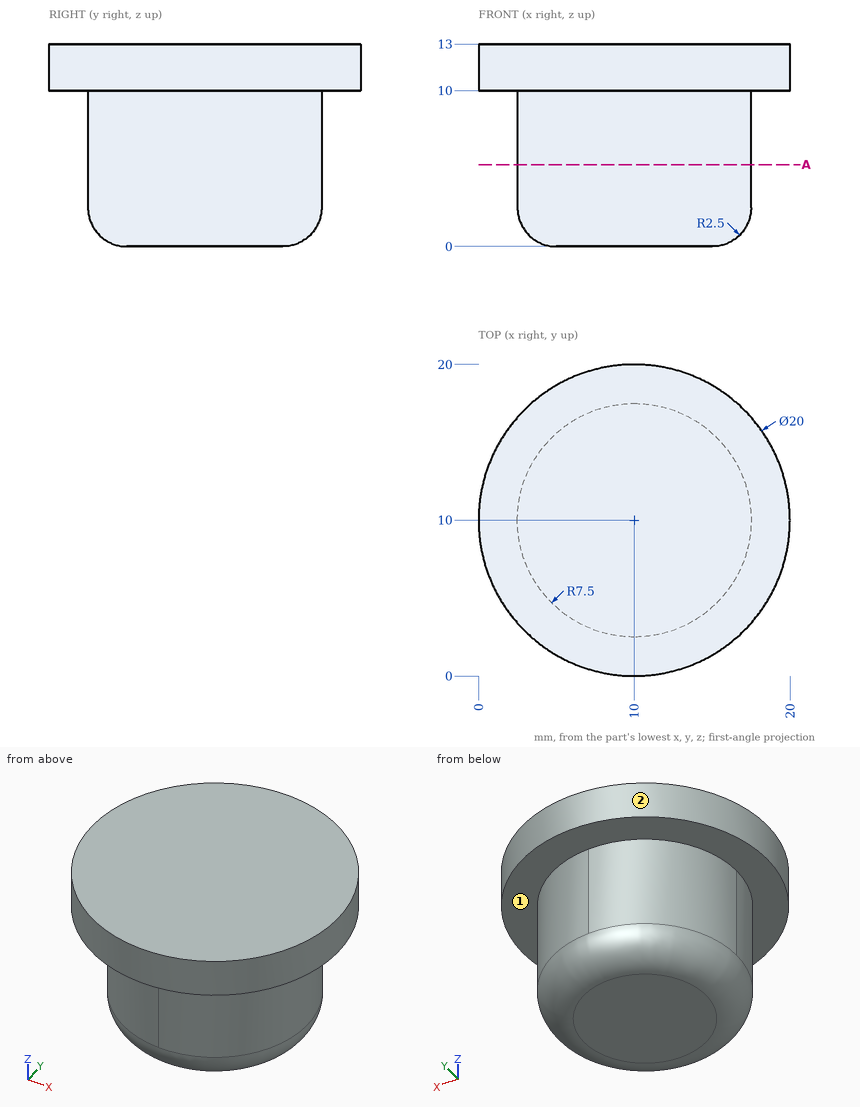
Job drawing, mm, ordinate dimensions from the low corner. One solid piece. A direction names the side the tool comes from. Coordinates: 2 decimals unless noted, no trailing zeros. Write each loop counter-clockwise with the first axis right and the second up, starting at its lowest first coordinate (ties: lowest second). Pieces come first, ordered by that corner, then holes.
Item 1: Which spindle directions (+Z, -Z, +X, -X, +Y, -Y) get a long thin tool onto all of the face, cutting with end or side? Do the marked faces 1 and 2. Say none if no direction does.
Item 2: Probe line 1 (Z direction, x = 8.25, y = 1.5); line 2 (Z direction, x = 8.5, y = 4); line 3 (Y direction, x = 14.5, z = 0.5). List the from-to ranges inside material, lowest first.
Item 3: Pin check, flat tips, straight feed: pin 1 (1 mm diameter, centred on y = 18, z = 2, fed in from -X); pin 2 (5 mm diameter, centred on x = 4, z = 10, fed in from +Y); pin 3 (1 mm diameter, centred on y = 5.5, z = 7, fed in from -X); pin 4 (3 mm diameter, centred on x = 9, z = 1.5, fed in from -Y). Stop position of each tip, or through.
Item 4: Slice it at A-A (z = 5.25). Write the cut outline in (x, y).
Results found:
1. face 1: -Z
1. face 2: +Z, -Z
2. line 1: z = 10 to 13
2. line 2: z = 0.3 to 13
2. line 3: y = 5.31 to 14.69
3. pin 1: passes through
3. pin 2: stops at y = 19.37
3. pin 3: stops at x = 3.66
3. pin 4: stops at y = 2.5
4. outline: circle Ø15 at (10, 10)
